CAD build for the part. Positions are in the model's coordinates, mm. A direction names the side the tool comes from. Coordinates: 2 decimals unless noted, no trailing zeros. Loops run counter-clockwise (first coordinate to the right, second up) from the corner with the lowest first, then second, coordinate; pieces in that order, holes last. Notation, with made-up numbers: (21, 89.25) - (33, 89.25) arc R32 ccw to (33, 127.25) - close; hole circle Ø7 at (3, 85.5). An arc over 180 degrees is marked (long way). Put each result on its own line as item: value.
```python
from build123d import *

# Parameters (mm, degrees)
SKETCH1_W                               = 120.00000003
SKETCH1_H                               = 92.999999928
BOSS_EXTRUDE1_DEPTH                     = 6.35
AC_INLET_DEPTH                          = 152.951711059
AC_INLET_SCREWS_D                       = 2.2606
FUSEHOLDER_D                            = 13
POWER_SWITCH_R                          = 7.62
POWER_SWITCH_INLAY_DEPTH                = 3.175
POWER_SWITCH_3_R                        = 2.4892
POWER_SWITCH_HOLE_DEPTH                 = 152.951711059
POWER_START                             = -3.175
POWER_SWITCH_LOCK_TAB_DEPTH             = 2.286
LED_PANEL_MOUNT_D                       = 8.0264
ADVANCEDHOLE1_START                     = 3.175
ADVANCEDHOLE1_OUTLINE_R                 = 17.4625
ADVANCEDHOLE1_DEPTH                     = 3.175
ADVANCEDHOLE1_2_OUTLINE_R               = 10.922
ADVANCEDHOLE1_2_DEPTH                   = 3.175
CBORE_FOR_M8_HEX_HEAD_BOLT2_D           = 8.4
CBORE_FOR_M8_HEX_HEAD_BOLT2_CBORE_D     = 18.01
CBORE_FOR_M8_HEX_HEAD_BOLT2_CBORE_DEPTH = 2.54
F_4_40_TAPPED_HOLE1_D                   = 2.2606
F_4_40_TAPPED_HOLE1_DEPTH               = 8.8646
F_4_40_TAPPED_HOLE1_TIP                 = 0.679152758
F_4_40_TAPPED_HOLE2_D                   = 2.2606
F_4_40_TAPPED_HOLE2_DEPTH               = 8.8646
F_4_40_TAPPED_HOLE2_TIP                 = 0.679152758
F_4_40_TAPPED_HOLE4_D                   = 2.2606
F_4_40_TAPPED_HOLE4_DEPTH               = 8.8646
F_4_40_TAPPED_HOLE4_TIP                 = 0.679152758


# Read off the part's stored shape, not the designer's step: AdvancedHole1, #4-40 Tapped Hole3
with BuildPart() as part:
    # Sketch1 → Boss-Extrude1 (new body)
    with BuildSketch(Plane.XY):
        with Locations((60.000000015, 46.499999964)):
            Rectangle(SKETCH1_W, SKETCH1_H)
    extrude(amount=BOSS_EXTRUDE1_DEPTH)

    # Sketch6 → AC Inlet (cut, through all)
    with BuildSketch(Plane(origin=(0, 0, 0), x_dir=(-1, 0, 0), z_dir=(0, 0, -1))):
        with BuildLine():
            Line((-51.435, 35.814), (-27.305, 35.814))
            ThreePointArc((-27.305, 35.814), (-25.05993597, 34.88406403), (-24.13, 32.639))
            Line((-24.13, 32.639), (-24.13, 18.161))
            ThreePointArc((-24.13, 18.161), (-25.05993597, 15.91593597), (-27.305, 14.986))
            Line((-27.305, 14.986), (-51.435, 14.986))
            ThreePointArc((-51.435, 14.986), (-53.68006403, 15.91593597), (-54.61, 18.161))
            Line((-54.61, 18.161), (-54.61, 32.639))
            ThreePointArc((-54.61, 32.639), (-53.68006403, 34.88406403), (-51.435, 35.814))
        make_face()
    extrude(amount=-AC_INLET_DEPTH, mode=Mode.SUBTRACT)

    # AC Inlet Screws (through all)
    with Locations(Plane(origin=(0, 0, 0), x_dir=(-1, 0, 0), z_dir=(0, 0, -1))):
        with Locations((-59.3725, 25.4), (-19.3675, 25.4)):
            Hole(AC_INLET_SCREWS_D / 2)

    # Fuseholder (through all)
    with Locations(Plane(origin=(0, 0, 0), x_dir=(-1, 0, 0), z_dir=(0, 0, -1))):
        with Locations((-78.4225, 25.4)):
            Hole(FUSEHOLDER_D / 2)

    # Power Switch → Power Switch Inlay (cut)
    with BuildSketch(Plane.XY.offset(6.35)):
        with Locations((100.0125, 25.4)):
            Circle(POWER_SWITCH_R)
    extrude(amount=-POWER_SWITCH_INLAY_DEPTH, mode=Mode.SUBTRACT)

    # Power Switch<3> → Power Switch Hole (cut, through all)
    with BuildSketch(Plane.XY.offset(6.35)):
        with Locations((100.0125, 25.4)):
            Circle(POWER_SWITCH_3_R)
    extrude(amount=-POWER_SWITCH_HOLE_DEPTH, mode=Mode.SUBTRACT)

    # Power Switch<4> → Power Switch Lock Tab (cut)
    with BuildSketch(Plane.XY.offset(6.35).offset(POWER_START)):
        with BuildLine():
            Line((99.7585, 20.2525), (100.2665, 20.2525))
            ThreePointArc((100.2665, 20.2525), (101.219, 19.3), (100.2665, 18.3475))
            Line((100.2665, 18.3475), (99.7585, 18.3475))
            ThreePointArc((99.7585, 18.3475), (98.806, 19.3), (99.7585, 20.2525))
        make_face()
    extrude(amount=-POWER_SWITCH_LOCK_TAB_DEPTH, mode=Mode.SUBTRACT)

    # LED Panel Mount (through all)
    with Locations(Plane(origin=(0, 0, 0), x_dir=(-1, 0, 0), z_dir=(0, 0, -1))):
        with Locations((-31.75, 68.869999928)):
            Hole(LED_PANEL_MOUNT_D / 2)

    # AdvancedHole1 outline → AdvancedHole1 (cut)
    with BuildSketch(Plane.XY.offset(ADVANCEDHOLE1_START)):
        with Locations((81.90000003, 56.169999928)):
            Circle(ADVANCEDHOLE1_OUTLINE_R)
    extrude(amount=ADVANCEDHOLE1_DEPTH, mode=Mode.SUBTRACT)

    # AdvancedHole1 2 outline → AdvancedHole1 2 (cut)
    with BuildSketch(Plane.XY):
        with Locations((81.90000003, 56.169999928)):
            Circle(ADVANCEDHOLE1_2_OUTLINE_R)
    extrude(amount=ADVANCEDHOLE1_2_DEPTH, mode=Mode.SUBTRACT)

    # CBORE for M8 Hex Head Bolt2 (through all)
    with Locations(Plane.XY.offset(6.35)):
        with Locations((31.75, 68.869999928)):
            CounterBoreHole(CBORE_FOR_M8_HEX_HEAD_BOLT2_D / 2, CBORE_FOR_M8_HEX_HEAD_BOLT2_CBORE_D / 2, CBORE_FOR_M8_HEX_HEAD_BOLT2_CBORE_DEPTH)

    # #4-40 Tapped Hole1
    with Locations(Plane(origin=(0, 0, 0), x_dir=(-1, 0, 0), z_dir=(0, -1, 0))):
        with Locations((-24.000000006, -3.175), (-96.000000024, -3.175)):
            Hole(F_4_40_TAPPED_HOLE1_D / 2, depth=F_4_40_TAPPED_HOLE1_DEPTH)
            with Locations((0, 0, -(F_4_40_TAPPED_HOLE1_DEPTH + F_4_40_TAPPED_HOLE1_TIP / 2))):  # 118° drill point
                Cone(0, F_4_40_TAPPED_HOLE1_D / 2, F_4_40_TAPPED_HOLE1_TIP, mode=Mode.SUBTRACT)

    # #4-40 Tapped Hole2
    with Locations(Plane(origin=(0, 92.999999928, 0), x_dir=(1, 0, 0), z_dir=(0, 1, 0))):
        with Locations((24.000000006, -3.175), (96.000000024, -3.175)):
            Hole(F_4_40_TAPPED_HOLE2_D / 2, depth=F_4_40_TAPPED_HOLE2_DEPTH)
            with Locations((0, 0, -(F_4_40_TAPPED_HOLE2_DEPTH + F_4_40_TAPPED_HOLE2_TIP / 2))):  # 118° drill point
                Cone(0, F_4_40_TAPPED_HOLE2_D / 2, F_4_40_TAPPED_HOLE2_TIP, mode=Mode.SUBTRACT)

    # #4-40 Tapped Hole3 outline → #4-40 Tapped Hole3 (revolve, cut)
    with BuildSketch(Plane(origin=(0, 23.249999982, 3.175), x_dir=(0, 1, 0), z_dir=(0, 0, -1))):
        Polygon((1.1303, 8.8646), (0, 9.543752758), (0, 0), (1.1303, 0), align=None)
    revolve(axis=Axis((0, 23.249999982, 3.175), (1, 0, 0)), mode=Mode.SUBTRACT)

    # 4-40 Tapped Hole3 2 outline → 4-40 Tapped Hole3 2 (revolve, cut)
    with BuildSketch(Plane(origin=(0, 69.749999946, 3.175), x_dir=(0, 1, 0), z_dir=(0, 0, -1))):
        Polygon((1.1303, 8.8646), (0, 9.543752758), (0, 0), (1.1303, 0), align=None)
    revolve(axis=Axis((0, 69.749999946, 3.175), (1, 0, 0)), mode=Mode.SUBTRACT)

    # #4-40 Tapped Hole4
    with Locations(Plane(origin=(120.00000003, 0, 0), x_dir=(0, 0, -1), z_dir=(1, 0, 0))):
        with Locations((-3.175, 69.749999946), (-3.175, 23.249999982)):
            Hole(F_4_40_TAPPED_HOLE4_D / 2, depth=F_4_40_TAPPED_HOLE4_DEPTH)
            with Locations((0, 0, -(F_4_40_TAPPED_HOLE4_DEPTH + F_4_40_TAPPED_HOLE4_TIP / 2))):  # 118° drill point
                Cone(0, F_4_40_TAPPED_HOLE4_D / 2, F_4_40_TAPPED_HOLE4_TIP, mode=Mode.SUBTRACT)


solid = part.part
```
Q1. Mould opens along X. For faces 1 (the flat face through (0, 46, 3)), 2 (the flat face through (59, 47, 0)), 3 (the cylindrical face through (35.905, 60.881, 5.098)), 4 (the flat face through (120, 46, 3)) say: +X half, -X half, draft (parallel to the pull), parting line (faces both ways), or undercut.
Determined:
face 1: -X half
face 2: draft
face 3: undercut
face 4: +X half
Q2. Slice it at A-A, the plane x = 31.75. Give the cut face in (y, z) (3 decimals), then the cut area to 3 significant figures.
Determined:
outline: (0, 0) - (14.986, 0) - (14.986, 6.35) - (0, 6.35) - close; (35.814, 0) - (64.67, 0) - (64.67, 3.81) - (59.865, 3.81) - (59.865, 6.35) - (35.814, 6.35) - close; (73.07, 0) - (93, 0) - (93, 6.35) - (77.875, 6.35) - (77.875, 3.81) - (73.07, 3.81) - close
area: 381 mm2
Q3. Pin check, flat tips, straight feed: pin 1 Ø1.8 at (x, z) = (96, 3.175) entering from +Y; pin 2 Ø1.8 at (y, z) = (23.25, 3.175) entering from +X; pin 3 Ø17.5 at (x, y) = (87, 57.5) entering from +Z (3 decimals). Stop position of each tip, or through.
Determined:
pin 1: y = 84
pin 2: x = 111
pin 3: z = 3.175
Q4. Tool access for faces 5 (the cylindrical face through (92.4, 25.7, 4.8)), 6 (the flat face through (59, 93, 3)), 7 (the flat face through (24.13, 26, 3)): list every direction of +Z, -Z, +X, -X, +Y, -Y with a clear straight run to the whole face (end or side of a thin tool).
Determined:
face 5: +Z
face 6: +Z, -Z, +X, -X, +Y
face 7: +Z, -Z
Q5. Slice it at C-C, the plane x = 77. Give the cut face in (y, z) (3 decimals).
Determined:
outline: (0, 0) - (19.058, 0) - (19.058, 6.35) - (0, 6.35) - close; (31.742, 0) - (46.409, 0) - (46.409, 3.175) - (39.409, 3.175) - (39.409, 6.35) - (31.742, 6.35) - close; (65.931, 0) - (93, 0) - (93, 6.35) - (72.931, 6.35) - (72.931, 3.175) - (65.931, 3.175) - close
Q6. Wall check: L1, parallel to Y at x = 115, z = 3; L2, parallel to X at y = 24.5, z = 1.5; L3, parallel to X at y = 56.5, z = 2.25. Give the ranges that are in metal, low to high. Write a range as from..to.
Determined:
L1: 0..22.13, 24.37..68.63, 70.87..93
L2: 0..18.68, 20.05..24.13, 54.61..58.69, 60.06..71.99, 84.86..97.69, 102.33..120
L3: 0..70.98, 92.82..120
